Autodesk Inventor part; units mm, degrees
ref_plane "YZ Plane" through (0, 0, 0) normal (1, 0, 0) x (0, 1, 0)
ref_plane "XZ Plane" through (0, 0, 0) normal (0, 1, 0) x (-1, 0, 0)
ref_plane "XY Plane" through (0, 0, 0) normal (0, 0, 1) x (1, 0, 0)
sketch "Skizze1" plane through (0, 0, 0) normal (0, 0, 1) x (1, 0, 0)
  line L0 (0, 0) -> (166, 0)
  line L1 (166, 0) -> (166, 80)
  line L2 (166, 80) -> (0, 80)
  line L3 (0, 80) -> (0, 0)
  dimension "d0" = 80
  dimension "d1" = 166
extrude "Extrusion1" add sketch "Skizze1" along normal blind 2
sketch "Skizze2" plane through (0, 0, 2) normal (0, 0, 1) x (1, 0, 0)
  line L0 (0, 80) -> (0, 0)
  line L1 (166, 0) -> (166, 80)
  line L2 (0, 0) -> (166, 0)
  line L3 (166, 0) -> (166, 80)
  line L4 (166, 80) -> (0, 80)
  line L5 (0, 80) -> (0, 0)
  line L6 (2, 78) -> (164, 78)
  line L7 (164, 78) -> (164, 2)
  line L8 (164, 2) -> (2, 2)
  line L9 (2, 2) -> (2, 78)
  dimension "d4" = 2
  dimension "d6" = 2
  dimension "d7" = 2
  dimension "d8" = 2
extrude "Extrusion2" add sketch "Skizze2" along normal blind 65
sketch "Skizze4" plane through (0, 0, 2) normal (0, 0, 1) x (1, 0, 0)
  line L0 (2, 2) -> (2, 78)
  line L1 (164, 2) -> (2, 2)
  line L2 (2, 78) -> (164, 78)
  line L3 (164, 78) -> (164, 2)
  line L4 (164, 2) -> (2, 2)
  line L5 (2, 2) -> (2, 78)
  line L6 (2, 68) -> (12, 68)
  line L7 (12, 68) -> (12, 78)
  line L8 (12, 78) -> (2, 78)
  line L9 (2, 78) -> (2, 68)
  line L10 (2, 2) -> (12, 2)
  line L11 (12, 2) -> (12, 12)
  line L12 (12, 12) -> (2, 12)
  line L13 (2, 12) -> (2, 2)
  line L14 (164, 78) -> (164, 2)
  line L15 (2, 78) -> (164, 78)
  line L16 (164, 68) -> (154, 68)
  line L17 (154, 68) -> (154, 78)
  line L18 (154, 78) -> (164, 78)
  line L19 (164, 78) -> (164, 68)
  line L20 (164, 2) -> (154, 2)
  line L21 (154, 2) -> (154, 12)
  line L22 (154, 12) -> (164, 12)
  line L23 (164, 12) -> (164, 2)
  point P0 (0, 0)
  point P1 (164, 12)
  point P2 (12, 2)
  point P3 (2, 68)
  dimension "d20" = 10
  dimension "d21" = 10
  dimension "d22" = 10
  dimension "d23" = 10
  dimension "d41" = 10
  dimension "d55" = 10
extrude "Extrusion3" add sketch "Skizze4" along normal blind 50 contours L0 L12 L11 L1 | L0 L2 L7 L6 | L21 L22 L3 L1 | L2 L3 L16 L17
sketch "Skizze5" plane through (0, 0, 2) normal (0, 0, 1) x (1, 0, 0)
  line L0 (2, 78) -> (164, 78)
  line L1 (2, 2) -> (2, 78)
  line L2 (2, 53) -> (7, 53)
  line L3 (7, 53) -> (7, 49)
  line L4 (7, 49) -> (2, 49)
  line L5 (2, 49) -> (2, 53)
  line L6 (2, 38) -> (7, 38)
  line L7 (7, 38) -> (7, 34)
  line L8 (7, 34) -> (2, 34)
  line L9 (2, 34) -> (2, 38)
  line L10 (164, 49) -> (159, 49)
  line L11 (159, 49) -> (159, 53)
  line L12 (159, 53) -> (164, 53)
  line L13 (164, 53) -> (164, 49)
  line L14 (164, 78) -> (164, 2)
  line L15 (164, 34) -> (159, 34)
  line L16 (159, 34) -> (159, 38)
  line L17 (159, 38) -> (164, 38)
  line L18 (164, 38) -> (164, 34)
  point P0 (0, 0)
  point P1 (2, 34)
  point P2 (2, 49)
  dimension "d30" = 11
  dimension "d31" = 4
  dimension "d32" = 4
  dimension "d33" = 5
  dimension "d34" = 25
  dimension "d37" = 5
  dimension "d38" = 0
  dimension "d58" = 25
  dimension "d59" = 4
  dimension "d60" = 11
extrude "Extrusion4" add sketch "Skizze5" along normal blind 50
sketch "Skizze3" plane through (0, 0, 0) normal (-1, 0, 0) x (0, 0, 1)
  line L0 (0, 80) -> (67, 80)
  line L1 (52, 12) -> (2, 12)
  line L2 (2, 34) -> (52, 34)
  line L3 (2, 34) -> (2, 12)
  point P0 (0, 0)
  point P1 (47, 23)
  point P2 (67, 12)
  point P3 (67, 34)
  dimension "d52" = 11
  dimension "d53" = 11
  dimension "d54" = 45
hole "Bohrung1" at (0, 23, 47) direction (1, 0, 0) diameter 20 depth 8 tip angle 118
sketch "Skizze6" plane through (0, 0, 52) normal (0, 0, 1) x (1, 0, 0)
  line L0 (4.15, 76.15) -> (9.85, 76.15)
  line L1 (9.85, 76.15) -> (9.85, 69.85)
  line L2 (9.85, 69.85) -> (4.15, 69.85)
  line L3 (4.15, 69.85) -> (4.15, 76.15)
  line L4 (2, 2) -> (2, 78)
  line L5 (2, 68) -> (12, 68)
  line L6 (4.15, 10.15) -> (9.85, 10.15)
  line L7 (9.85, 10.15) -> (9.85, 3.85)
  line L8 (9.85, 3.85) -> (4.15, 3.85)
  line L9 (4.15, 3.85) -> (4.15, 10.15)
  line L10 (12, 12) -> (2, 12)
  line L11 (156.15, 76.15) -> (161.85, 76.15)
  line L12 (161.85, 76.15) -> (161.85, 69.85)
  line L13 (161.85, 69.85) -> (156.15, 69.85)
  line L14 (156.15, 69.85) -> (156.15, 76.15)
  line L15 (154, 78) -> (154, 68)
  line L16 (156.15, 10.15) -> (161.85, 10.15)
  line L17 (161.85, 10.15) -> (161.85, 3.85)
  line L18 (161.85, 3.85) -> (156.15, 3.85)
  line L19 (156.15, 3.85) -> (156.15, 10.15)
  line L20 (2, 78) -> (164, 78)
  point P0 (0, 0)
  dimension "d42" = 5.7
  dimension "d43" = 6.3
  dimension "d44" = 2.15
  dimension "d45" = 1.85
  dimension "d46" = 6.3
  dimension "d47" = 1.85
  dimension "d48" = 5.7
  dimension "d49" = 2.15
  dimension "d56" = 1.85
  dimension "d57" = 6.3
extrude "Extrusion5" cut sketch "Skizze6" against normal blind 3
properties part number "TimBoden"
Work out the finished part from the listing and answer in its coordinate system (mm). A direction names the side the tool comes from. Coordinates: 2 decimals unless noted, no trailing zeros. Write each loop counter-clockwise with the first axis right and the second up, starting at its lowest first coordinate (ties: lowest second). Pieces come first, ordered by that corner, then holes. Notation, with made-up numbers: (9.25, 19.5) - (57.25, 19.5) arc R25 ccw to (57.25, 45.5) - close; hole circle Ø3 at (6, 87.5). An arc over 180 degrees is marked (long way). Answer as a JSON object with one key per item and string values.
Q1. Find section A-A (y = 23). Write down the section's boundary in (x, z).
Results list:
{"outline": "(0, 0) - (166, 0) - (166, 67) - (164, 67) - (164, 2) - (2, 2) - (2, 37) - (0, 37) - close; (0, 57) - (2, 57) - (2, 67) - (0, 67) - close"}
Q2. Find section D-D (x = 141). Write down the section's boundary in (y, z).
Results list:
{"outline": "(0, 0) - (80, 0) - (80, 67) - (78, 67) - (78, 2) - (2, 2) - (2, 67) - (0, 67) - close"}
Q3. Consider L1, parallel to Y at x = 1.05, z = 47; L2, parallel to X at y = 26, z = 19; L3, parallel to Y at x = 45, z = 26. Determine where each line is inside the solid, lowest interval first. Write a range as from..to.
Results list:
{"L1": "y = 0..13, 33..80", "L2": "x = 0..2, 164..166", "L3": "y = 0..2, 78..80"}
Q4. Find section C-C (y = 71.5). Write down the section's boundary in (x, z), plus the area to 3 significant figures.
Results list:
{"outline": "(0, 0) - (166, 0) - (166, 67) - (164, 67) - (164, 52) - (161.85, 52) - (161.85, 49) - (156.15, 49) - (156.15, 52) - (154, 52) - (154, 2) - (12, 2) - (12, 52) - (9.85, 52) - (9.85, 49) - (4.15, 49) - (4.15, 52) - (2, 52) - (2, 67) - (0, 67) - close", "area": "1,560 mm^2"}
Q5. Which of the six approach directions +Z, -Z, +X, -X, +Y, -Y give full straight-line access (tool end or side, diameter ignored) to faces 1 (the flat face through (166, 39, 33)), 2 (the flat face through (7, 51, 27))?
Results list:
{"face 1": "+Z, -Z, +X, +Y, -Y", "face 2": "+Z"}
Q6. For a pull along Y with two mould halves and no side action, classify faces 3 (the flat face through (82, 0, 33)), 4 (the flat face through (82, 41, 0)), 5 (the flat face through (161, 51, 52)) as pulls with the +Y half, pulls with the -Y half, needs draft (parallel to the pull), parting line crosses it, or undercut.
Results list:
{"face 3": "pulls with the -Y half", "face 4": "needs draft", "face 5": "undercut"}
Q7. Given pin 1 Ø12 at (x, y) = (89.5, 35) entering from +Z; pin 2 Ø1.2 at (x, y) = (161, 50.5) entering from +Z; pin 3 Ø1.7 at (x, y) = (8, 73) entering from +Z, each flat-ended and moving along its own axis, determine where each tip first touches the part or whether it passes through.
Results list:
{"pin 1": "stops at z = 2", "pin 2": "stops at z = 52", "pin 3": "stops at z = 49"}
